```python
from build123d import *

# Parameters (mm, degrees)
PAD_DEPTH    = 1.24
SKETCH001_W  = 12.1
SKETCH001_H  = 37.2
PAD001_DEPTH = 1.24


with BuildPart() as part:
    # Sketch → Pad (new body)
    with BuildSketch(Plane.XY):
        with BuildLine():
            add(Edge.make_bspline(
                [(0, 16.665), (-20.091789, 16.665), (-10.045895, -8.3325), (0, -33.33), (10.045895, -8.3325), (20.091789, 16.665), (0, 16.665)],
                knots=[0, 0, 0, 2.094395, 2.094395, 4.18879, 4.18879, 6.283185, 6.283185, 6.283185], degree=2, weights=[1, 0.5, 1, 0.5, 1, 0.5, 1]))
        make_face()
    extrude(amount=PAD_DEPTH)

    # Sketch001 (on Face2 of Pad) → Pad001 (join)
    with BuildSketch(Plane(origin=(0, 0, 0), x_dir=(1, 0, 0), z_dir=(0, 0, -1))):
        Rectangle(SKETCH001_W, SKETCH001_H)
    extrude(amount=-PAD001_DEPTH)


solid = part.part
```
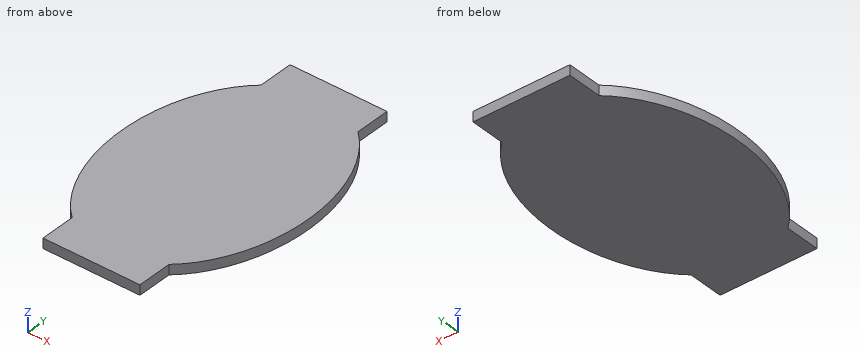
Geometry: final body of the model. Coordinates: model frame, mm. Round coordinates to 2 decimals unless told otherwise and drop trailing zeros. Loops run counter-clockwise (first coordinate to the right, second up) from the corner with the lowest first, then second, coordinate; pieces in that order, holes last.
Item 1: Line query: L1, parallel to X at y = -15, z = 1.1; L2, parallel to Y at x = 6.5, z = 0.4. Output: solid intervals per line, ascending.
Checked values:
L1: x = -6.05 to 6.05
L2: y = -13.8 to 13.8
Item 2: Section A-A, the plane y = 16. Output: boundary loops of the cut face in (x, z), plus the area to 3 significant figures.
Checked values:
outline: (-6.05, 0) - (6.05, 0) - (6.05, 1.24) - (-6.05, 1.24) - close
area: 15.0 mm2
Item 3: Contact query for flat-ended pins moving along their axis: P1, Ø0.6, axis at y = -15.5, z = 0.5, coming from the +X side; P2, Ø0.6, axis at y = -16.5, z = 0.5, coming from the -X side. Output: stop coordinate, or through.
Checked values:
P1: stops at x = 6.05
P2: stops at x = -6.05
